Geometry: final body of the model. Coordinates: model frame, mm. A direction names the side the tool comes from. Give positions to 0.01 mm unless a question says otherwise; leave off trailing zeros. Write each loop counter-clockwise with the first axis right and the second up, starting at its lowest first coordinate (ties: lowest second). Pieces come first, ordered by that corner, then holes.
Q1. Section B-B (x = 3.1). Return the cut outline in (y, z).
Q2. Section C-C (y = 3.1). Return the cut outline in (x, z).
Q3. Line query: line 1 (Z direction, x = 4, y = 2); line 2 (Z direction, x = 6, y = 5.5); line 3 (Y direction, x = 5.25, z = 6.5). Output: solid intervals per line, ascending.
Q4. Reachability of faces 1 (the flat face through (0.7, 5.4, -0.3)), 2 (the cylindrical face through (4.49, 2.04, -0.49)) from +Z, -Z, +X, -X, +Y, -Y: full face, straight path, thin tool, end or side. Return the list, or none.
Q5. Section A-A (z = 5.5). Return the cut outline in (x, y).
Q6. Mould query, pull axis Y, two halves, no side actions, for faces 3 (the flat face through (5.4, 0.7, -0.3)), 4 (the flat face through (3, 0, 2)), 5 (the flat face through (2, 5, 0)). Classes: +Y half, -Y half, draft (parallel to the pull), parting line (faces both ways), or undercut.
Q7. Pin query (flat end, axial travel): pin 1 Ø0.5 at (x, y) = (5.5, 5.5) entering from -Z; pin 2 Ø1.5 at (x, y) = (4, 4) entering from +Z. Return the tip coordinate at first contact, or that it passes through.
Q8. Section D-D (x = 0.75). Return the cut outline in (y, z), plus the area to 3 significant figures.
from build123d import *

# Parameters (mm, degrees)
CROQUIS1_W                 = 6.2
CROQUIS1_H                 = 6.2
SALIENTE_EXTRUIR1_DEPTH    = 3.5
CROQUIS2_W                 = 6.2
CROQUIS2_H                 = 0.1
CORTAR_EXTRUIR1_DEPTH      = 0.1
CORTAR_EXTRUIR2_DEPTH      = 10.375499987
CORTAR_EXTRUIR2_DEPTH_BACK = 10.375499987
CROQUIS3_W                 = 0.1
CROQUIS3_H                 = 0.1
CORTAR_EXTRUIR3_DEPTH      = 10.375499987
CORTAR_EXTRUIR3_DEPTH_BACK = 10.375499987
CROQUIS4_W                 = 0.1
CROQUIS4_H                 = 0.1
CROQUIS5_R                 = 1.75
SALIENTE_EXTRUIR2_DEPTH    = 1
CROQUIS6_R                 = 0.5
SALIENTE_EXTRUIR3_DEPTH    = 0.3
SALIENTE_EXTRUIR4_DEPTH    = 3.5


with BuildPart() as part:
    # Croquis1 → Saliente-Extruir1 (new body)
    with BuildSketch(Plane.XY):
        with Locations((3.1, 3.1)):
            Rectangle(CROQUIS1_W, CROQUIS1_H)
    extrude(amount=SALIENTE_EXTRUIR1_DEPTH)

    # Croquis2 → Cortar-Extruir1 (cut)
    with BuildSketch(Plane(origin=(0, 6.2, 0), x_dir=(1, 0, 0), z_dir=(0, 1, 0))):
        with Locations((3.1, -0.7)):
            Rectangle(CROQUIS2_W, CROQUIS2_H)
    extrude(amount=-CORTAR_EXTRUIR1_DEPTH, mode=Mode.SUBTRACT)

    # Croquis3 → Cortar-Extruir2 (cut, two sides: drawn at the far end of the back side and taken through both)
    with BuildSketch(Plane(origin=(0, 6.1, 0), x_dir=(1, 0, 0), z_dir=(0, 1, 0)).offset(-CORTAR_EXTRUIR2_DEPTH_BACK)):
        with Locations((0.05, -0.7)):
            Rectangle(CROQUIS3_W, CROQUIS3_H)
        with Locations((6.15, -0.7)):
            Rectangle(CROQUIS3_W, CROQUIS3_H)
    extrude(amount=CORTAR_EXTRUIR2_DEPTH + CORTAR_EXTRUIR2_DEPTH_BACK, mode=Mode.SUBTRACT)

    # Croquis4 → Cortar-Extruir3 (cut, two sides: drawn at the far end of the back side and taken through both)
    with BuildSketch(Plane.ZY.offset(-0.1).offset(-CORTAR_EXTRUIR3_DEPTH_BACK)):
        with Locations((0.7, 0.05)):
            Rectangle(CROQUIS4_W, CROQUIS4_H)
    extrude(amount=CORTAR_EXTRUIR3_DEPTH + CORTAR_EXTRUIR3_DEPTH_BACK, mode=Mode.SUBTRACT)

    # Croquis5 → Saliente-Extruir2 (add)
    with BuildSketch(Plane(origin=(0, 0, 0), x_dir=(-1, 0, 0), z_dir=(0, 0, -1))):
        with Locations((-3.1, 3.1)):
            Circle(CROQUIS5_R)
    extrude(amount=SALIENTE_EXTRUIR2_DEPTH)

    # Croquis6 → Saliente-Extruir3 (add)
    with BuildSketch(Plane(origin=(0, 0, 0), x_dir=(-1, 0, 0), z_dir=(0, 0, -1))):
        with Locations(Location((-0.75, 0.75, 0), (0, 0, 180))):
            Circle(CROQUIS6_R)
        with Locations(Location((-5.45, 0.75, 0), (0, 0, 180))):
            Circle(CROQUIS6_R)
        with Locations(Location((-0.75, 5.45, 0), (0, 0, 180))):
            Circle(CROQUIS6_R)
        with Locations(Location((-5.45, 5.45, 0), (0, 0, 180))):
            Circle(CROQUIS6_R)
    extrude(amount=SALIENTE_EXTRUIR3_DEPTH)

    # Croquis8 → Saliente-Extruir4 (add)
    with BuildSketch(Plane.XY.offset(3.5)):
        Polygon((5.6, 2.95), (5.6, 3.1), (5.6, 3.25), (5, 3.25), (5, 2.95), align=None)
        Polygon((0.6, 2.95), (0.6, 3.1), (0.6, 3.25), (1.2, 3.25), (1.2, 2.95), align=None)
    extrude(amount=SALIENTE_EXTRUIR4_DEPTH)


solid = part.part
Computed:
1. outline: (0, 0) - (1.35, 0) - (1.35, -1) - (4.85, -1) - (4.85, 0) - (6.2, 0) - (6.2, 0.65) - (6.1, 0.65) - (6.1, 0.75) - (6.2, 0.75) - (6.2, 3.5) - (0, 3.5) - (0, 0.75) - (0.1, 0.75) - (0.1, 0.65) - (0, 0.65) - close
2. outline: (0, 0) - (1.35, 0) - (1.35, -1) - (4.85, -1) - (4.85, 0) - (6.2, 0) - (6.2, 0.65) - (6.1, 0.65) - (6.1, 0.75) - (6.2, 0.75) - (6.2, 3.5) - (5.6, 3.5) - (5.6, 7) - (5, 7) - (5, 3.5) - (1.2, 3.5) - (1.2, 7) - (0.6, 7) - (0.6, 3.5) - (0, 3.5) - (0, 0.75) - (0.1, 0.75) - (0.1, 0.65) - (0, 0.65) - close
3. line 1: z = -1 to 3.5
3. line 2: z = 0 to 3.5
3. line 3: y = 2.95 to 3.25
4. face 1: -Z, +X, -X, +Y, -Y
4. face 2: -Z
5. outline: (0.6, 2.95) - (1.2, 2.95) - (1.2, 3.25) - (0.6, 3.25) - close; (5, 2.95) - (5.6, 2.95) - (5.6, 3.25) - (5, 3.25) - close
6. face 3: draft
6. face 4: -Y half
6. face 5: undercut
7. pin 1: stops at z = -0.3
7. pin 2: stops at z = 3.5
8. outline: (0, 0) - (0.25, 0) - (0.25, -0.3) - (1.25, -0.3) - (1.25, 0) - (4.95, 0) - (4.95, -0.3) - (5.95, -0.3) - (5.95, 0) - (6.2, 0) - (6.2, 0.65) - (6.1, 0.65) - (6.1, 0.75) - (6.2, 0.75) - (6.2, 3.5) - (3.25, 3.5) - (3.25, 7) - (2.95, 7) - (2.95, 3.5) - (0, 3.5) - (0, 0.75) - (0.1, 0.75) - (0.1, 0.65) - (0, 0.65) - close
8. area: 23.3 mm2
